```python
from build123d import *

# Parameters (mm, degrees)
F0_W     = 15
F0_H     = 15
F0_W_2   = 14
F0_H_2   = 14
F1_DEPTH = 60
F2_W     = 15
F2_H     = 6
F3_DEPTH = 0.01
F4_DEPTH = 60


with BuildPart() as f1:
    # F0 (on Top) → F1 (new body)
    with BuildSketch(Plane.XY):
        Rectangle(F0_W, F0_H)
        Rectangle(F0_W_2, F0_H_2, mode=Mode.SUBTRACT)
    extrude(amount=-F1_DEPTH)

    # F2 (on face) → F3 (join)
    with BuildSketch(Plane.YZ.offset(7.5)):
        with Locations((0, -7)):
            Rectangle(F2_W, F2_H)
    extrude(amount=F3_DEPTH)

    # F4 (add): a face of the model
    f4_faces = [f1.faces().sort_by_distance(p)[0] for p in [
        (0, -7.2878679656, -60),
    ]]
    extrude(f4_faces, amount=F4_DEPTH)


solid = f1.part
```
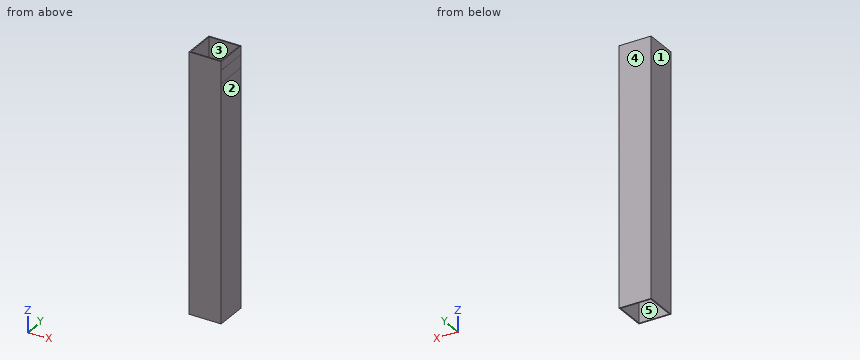
Input: part model. Units: mm. Frame: model coordinates. Face numbers are marked on the shaded views. A direction names the side the tool comes from. Coordinates: 2 decimals unless noted, no trailing zeros. Order: outer loops, then holes, each group sorted by start corner. A loop starts at its lowest first (then second) coordinate and runs counter-clockwise, first axis right, second up. Notation, with made-up numbers: (-28, 57) - (7, 57) arc R27 cw to (7, 90) - close; hole circle Ø8 at (-32, 54). An arc over 180 degrees is marked (long way). Put each result on its own line as item: value.
1. Cut plane C-C on z = -36. Return the cut outline in (x, y).
Report:
outline: (-7.5, -7.5) - (7.5, -7.5) - (7.5, 7.5) - (-7.5, 7.5) - close; hole (-7, -7) - (7, -7) - (7, 7) - (-7, 7) - close
2. Reachability of the marked faces 4 and 5 from +Z, -Z, +X, -X, +Y, -Y: full face, straight path, thin tool, end or side. Return the list, or none.
Report:
face 4: +Z, -Z, +X, -X, +Y
face 5: +Z, -Z
3. Cut plane B-B on x = -1.5. Return the cut outline in (y, z), then the cut area to 3 significant figures.
Report:
outline: (-7.5, -120) - (-7, -120) - (-7, 0) - (-7.5, 0) - close; (7, -120) - (7.5, -120) - (7.5, 0) - (7, 0) - close
area: 120 mm2
4. Draft query along X for the marked faces 1, 2 and 3. Return one class per face: pulls with the +X half, pulls with the -X half, needs draft (parallel to the pull), parting line crosses it, or undercut.
Report:
face 1: pulls with the -X half
face 2: pulls with the +X half
face 3: undercut
5. Line query: line 1 along Y through (x, z) = (1.5, -74). Output: solid intervals per line, ascending.
Report:
line 1: y = -7.5 to -7, 7 to 7.5
6. Contact query for a flat-ended pin moving along its axis: pin 1 Ø7.5 at (y, z) = (0, -61) entering from +X. Output: stop coordinate, or through.
Report:
pin 1: stops at x = 7.5
